Job drawing, mm, ordinate dimensions from the low corner. One solid piece. A direction names the side the tool comes from. Round coordinates to 2 decimals unless told otherwise and drop trailing zeros. Order: outer loops, then holes, each group sorted by start corner. A loop starts at its lowest first (then second) coordinate and runs counter-clockwise, first axis right, second up. Notation, with made-up numbers: (18.5, 28) -> (49.5, 28) arc R9 cw to (49.5, 38) -> close; hole circle Ø8 at (-38.5, -37.75). An arc over 180 degrees is marked (long way). Use CSV: the item, a comma, the result in double quotes.
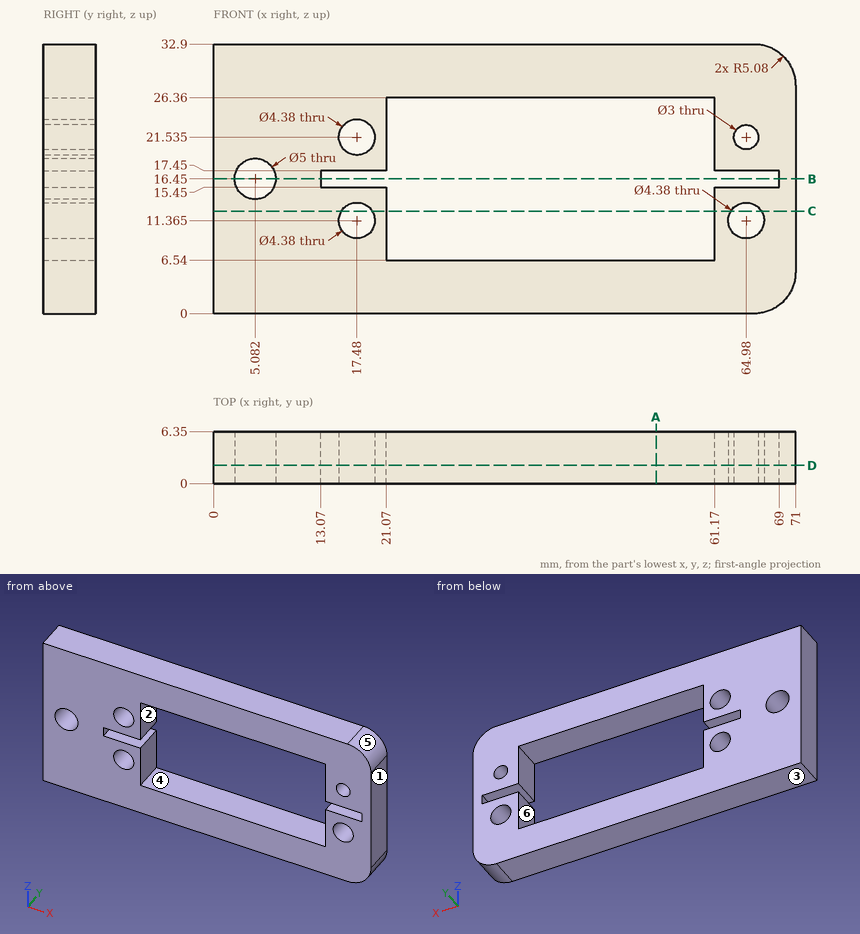
(1) Drop a flat-ended pin along its axis: P1, Ø4, axis at x = 64.98, z = 11.36, coming from the -Y side. Give the stop position or say it passes through.
Reply:
P1,"through"
(2) Probe probe 1 along X at (y, z) = (1, 24.5); probe 2 along Z at (x, y) = (53.5, 5.25); probe 3 along Z at (x, y) = (18, 3.5). List the from-to ranges inside material, lowest first. Write a range as [from, to].
Reply:
probe 1,"[0, 21.07], [61.17, 71]"
probe 2,"[0, 6.54], [26.36, 32.9]"
probe 3,"[0, 9.24], [13.49, 15.45], [17.45, 19.41], [23.66, 32.9]"
(3) Pull direction X, two halves, no side cores. Call the marked faces 1, 2, 3 and 4: released by +X, released by -X, zero draft, split by the parting line, or undercut.
Reply:
face 1,"released by +X"
face 2,"undercut"
face 3,"zero draft"
face 4,"undercut"
(4) Cut at D-D, the plane y = 2.25. State how many separate pieces and enclosed holes the cut face has, then the cut area to 3 significant figures.
Reply:
separate pieces,"1"
enclosed holes,"6"
area,"1,430 mm2"
(5) Cut at A-A, the plane x = 54. Give the cut face in (y, z).
Reply:
outline,"(0, 0) -> (6.35, 0) -> (6.35, 6.54) -> (0, 6.54) -> close; (0, 26.36) -> (6.35, 26.36) -> (6.35, 32.9) -> (0, 32.9) -> close"
(6) Which spindle directions (+Z, -Z, +X, -X, +Y, -Y) get a long thin tool onto all of the face, cutting with end or side? Do the marked faces 5 and 6. Say none if no direction does.
Reply:
face 5,"+Z, +X, +Y, -Y"
face 6,"+Y, -Y"
(7) Cut at B-B, the plane z = 16.45. Give the cut face in (x, y).
Reply:
outline,"(0, 0) -> (2.58, 0) -> (2.58, 6.35) -> (0, 6.35) -> close; (7.58, 0) -> (13.07, 0) -> (13.07, 6.35) -> (7.58, 6.35) -> close; (69, 0) -> (71, 0) -> (71, 6.35) -> (69, 6.35) -> close"
(8) Cut at C-C, the plane z = 12.5. Give the cut face in (x, y).
Reply:
outline,"(0, 0) -> (15.61, 0) -> (15.61, 6.35) -> (0, 6.35) -> close; (19.35, 0) -> (21.07, 0) -> (21.07, 6.35) -> (19.35, 6.35) -> close; (61.17, 0) -> (63.11, 0) -> (63.11, 6.35) -> (61.17, 6.35) -> close; (66.85, 0) -> (71, 0) -> (71, 6.35) -> (66.85, 6.35) -> close"
